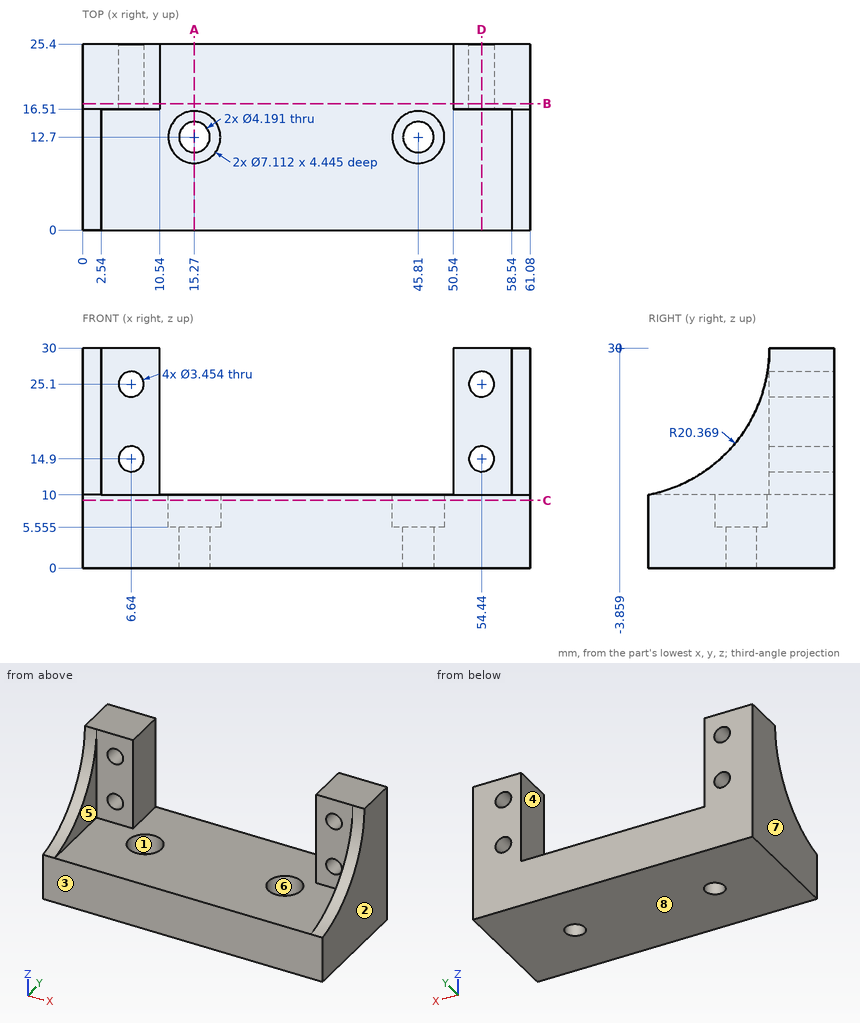
Job drawing, mm, ordinate dimensions from the low corner. One solid piece. A direction names the side the tool comes from. Round coordinates to 2 decimals unless told otherwise and drop trailing zeros. Write each loop counter-clockwise with the first axis right and the second up, starting at its lowest first coordinate (ties: lowest second). Pieces come first, ordered by that corner, then holes. Notation, with made-up numbers: M 36,45.5 L 42,45.5 A27 cw 42,80.5 Z; hole C -31,51.5 d2. An arc over 180 degrees is marked long. Return JSON: item names as keys, results as strings. Group by question number.
(1) Saw through at B-B on y = 17.25. Write the cut outline in (x, z) (1 decimal).
(2) Which spindle directions (+Z, -Z, +X, -X, +Y, -Y) get a long thin tool onto all of the face, cutting with end or side? Do the marked faces 4, 5, 6, 7 and 8. Say none if no direction does.
(3) Saw through at A-A on x = 15.27. Write the cut outline in (y, z) (1 decimal).
(4) Saw through at C-C on z = 9.25. Write the cut outline in (x, y).
(5) Pin check, flat tips, straight feed: pin 1 Ø4.5 at (x, z) = (54.44, 14.9) entering from +Y; pin 2 Ø3.5 at (x, y) = (14.5, 14.5) entering from +Z; pin 3 Ø5.5 at (x, y) = (45.81, 12.7) entering from +Z (3 decimals); pin 4 Ø9 at (x, z) = (53.5, 16.5) entering from -Y. Stop position of each tip, or through.
(6) Drill centre lines: probe 1 along Z at (x, y) = (6.64, 22); probe 2 along X at (y, z) = (23.5, 16.25) (1 decimal); probe 3 along Z at (x, y) = (20, 5.75). Where is each one in solid material? Low to high.
(7) Two-plate mould, pull along Y, no slides. Class the marked faces 1, 2 and 3: +Y half, -Y half, draft (parallel to the pull), parting line (faces both ways), or undercut.
(8) Saw through at D-D on x = 54.44. Write the cut outline in (y, z).
Returned:
{
 "1": {"outline": "M 0,0 L 61.1,0 L 61.1,30 L 50.5,30 L 50.5,10 L 10.5,10 L 10.5,30 L 0,30 Z; hole C 6.6,14.9 d3.5; hole C 6.6,25.1 d3.5; hole C 54.4,14.9 d3.5; hole C 54.4,25.1 d3.5"},
 "2": {"face 4": "+Z, +Y, -Y", "face 5": "+Z, -Y", "face 6": "+Z", "face 7": "+Z, -Z, -X, +Y, -Y", "face 8": "-Z, +X, -X, +Y, -Y"},
 "3": {"outline": "M 0,0 L 10.6,0 L 10.6,5.6 L 9.1,5.6 L 9.1,10 L 0,10 Z; M 14.8,0 L 25.4,0 L 25.4,10 L 16.3,10 L 16.3,5.6 L 14.8,5.6 Z"},
 "4": {"outline": "M 0,0 L 61.08,0 L 61.08,25.4 L 0,25.4 Z; hole C 15.27,12.7 d7.11; hole C 45.81,12.7 d7.11"},
 "5": {"pin 1": "y = 25.4", "pin 2": "z = 10", "pin 3": "z = 5.555", "pin 4": "y = 16.51"},
 "6": {"probe 1": "0 to 13.17, 16.63 to 23.37, 26.83 to 30", "probe 2": "0 to 5.6, 7.7 to 10.5, 50.5 to 53.4, 55.5 to 61.1", "probe 3": "0 to 10"},
 "7": {"face 1": "undercut", "face 2": "draft", "face 3": "-Y half"},
 "8": {"outline": "M 0,0 L 25.4,0 L 25.4,13.17 L 16.51,13.17 L 16.51,10 L 0,10 Z; M 16.51,16.63 L 25.4,16.63 L 25.4,23.37 L 16.51,23.37 Z; M 16.51,26.83 L 25.4,26.83 L 25.4,30 L 16.51,30 Z"}
}
